```python
from build123d import *

# Parameters (mm, degrees)
SKETCH1_W                  = 19.05
SKETCH1_H                  = 63.5
BOSS_EXTRUDE1_DEPTH        = 15.875
SKETCH2_R                  = 5.1435
CUT_EXTRUDE1_DEPTH         = 37.753282166
SKETCH3_R                  = 12.7
CUT_EXTRUDE2_DEPTH         = 3.96875
SKETCH4_R                  = 12.7
SKETCH4_R_2                = 7.9375
CUT_EXTRUDE3_DEPTH         = 0.79375
F_10_CLEARANCE_HOLE1_D     = 5.6134
F_10_CLEARANCE_HOLE1_DEPTH = 25.4
F_10_CLEARANCE_HOLE1_TIP   = 1.686435499
FILLET1_R                  = 1.5875
BOSS_EXTRUDE2_DEPTH        = 5.953125
FILLET3_R                  = 0.79375
FILLET4_R                  = 3.175


with BuildPart() as part:
    # Sketch1 → Boss-Extrude1 (new body)
    with BuildSketch(Plane.XY):
        Rectangle(SKETCH1_W, SKETCH1_H)
    extrude(amount=BOSS_EXTRUDE1_DEPTH)

    # Sketch2 → Cut-Extrude1 (cut, through all)
    with BuildSketch(Plane.XY.offset(15.875)):
        Circle(SKETCH2_R)
    extrude(amount=-CUT_EXTRUDE1_DEPTH, mode=Mode.SUBTRACT)

    # Sketch3 → Cut-Extrude2 (cut)
    with BuildSketch(Plane.XY.offset(15.875)):
        Circle(SKETCH3_R)
    extrude(amount=-CUT_EXTRUDE2_DEPTH, mode=Mode.SUBTRACT)

    # Sketch4 → Cut-Extrude3 (cut)
    with BuildSketch(Plane.XY.offset(11.90625)):
        Circle(SKETCH4_R)
        Circle(SKETCH4_R_2, mode=Mode.SUBTRACT)
    extrude(amount=-CUT_EXTRUDE3_DEPTH, mode=Mode.SUBTRACT)

    # #10 Clearance Hole1
    with Locations(Plane.XY.offset(15.875)):
        with Locations((0, 25.4), (0, -25.4)):
            Hole(F_10_CLEARANCE_HOLE1_D / 2, depth=F_10_CLEARANCE_HOLE1_DEPTH)
            with Locations((0, 0, -(F_10_CLEARANCE_HOLE1_DEPTH + F_10_CLEARANCE_HOLE1_TIP / 2))):  # 118° drill point
                Cone(0, F_10_CLEARANCE_HOLE1_D / 2, F_10_CLEARANCE_HOLE1_TIP, mode=Mode.SUBTRACT)

    # Fillet1
    fillet1_edges = [part.edges().sort_by_distance(p)[0] for p in [
        (9.525, -8.400260413, 13.49375),
        (-9.525, -8.400260413, 13.49375),
        (9.525, 8.400260413, 13.49375),
        (-9.525, 8.400260413, 13.49375),
        (-9.525, 0, 11.1125),
        (9.525, 0, 11.1125),
        (9.525, -31.75, 7.9375),
        (-9.525, -31.75, 7.9375),
    ]]
    fillet(fillet1_edges, radius=FILLET1_R - 0.0001)  # a hair under: the kernel refuses the full size

    # Sketch12 → Boss-Extrude2 (add)
    with BuildSketch(Plane(origin=(0, 0, 0), x_dir=(-1, 0, 0), z_dir=(0, 0, -1))):
        with BuildLine():
            Line((-15.875, 67.31), (-15.875, 51.435))
            Line((-15.875, 51.435), (-9.779, 51.435))
            Line((-9.779, 51.435), (-9.779, 54.61))
            ThreePointArc((-9.779, 54.61), (-6.604, 57.785), (-3.429, 54.61))
            Line((-3.429, 54.61), (-3.429, 45.085))
            Line((-3.429, 45.085), (-15.875, 45.085))
            Line((-15.875, 45.085), (-15.875, 31.75))
            Line((-15.875, 31.75), (-9.525, 3.175))
            Line((-9.525, 3.175), (-9.525, 31.75))
            Line((-9.525, 31.75), (9.525, 31.75))
            Line((9.525, 31.75), (9.525, 67.31))
            Line((9.525, 67.31), (-15.875, 67.31))
        make_face()
    extrude(amount=-BOSS_EXTRUDE2_DEPTH)

    # Fillet3
    fillet3_edges = [part.edges().sort_by_distance(p)[0] for p in [
        (9.779, 51.435, 2.9765625),
        (15.875, 51.435, 2.9765625),
        (9.525, 3.175, 2.9765625),
        (15.875, 31.75, 2.9765625),
        (15.875, 45.085, 2.9765625),
        (3.429, 45.085, 2.9765625),
    ]]
    fillet(fillet3_edges, radius=FILLET3_R)

    # Fillet4
    fillet4_edges = [part.edges().sort_by_distance(p)[0] for p in [
        (15.875, 67.31, 2.9765625),
        (-9.525, 67.31, 2.9765625),
    ]]
    fillet(fillet4_edges, radius=FILLET4_R)


with BuildPart() as body_2:
    # Mirror1: mirrored copy
    add(part.part.mirror(Plane.XY.offset(15.875)))


solid = body_2.part
```
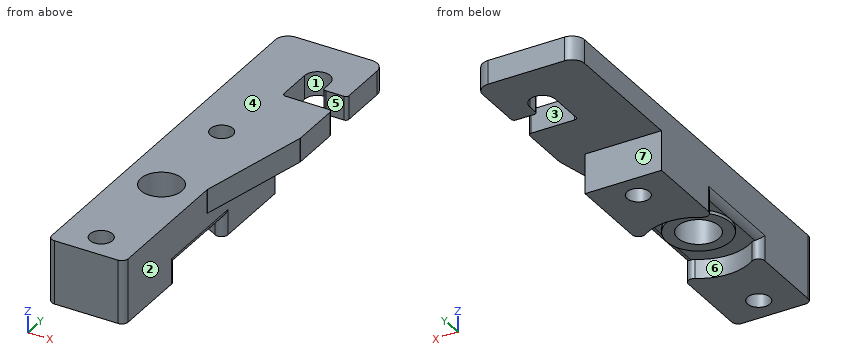
Design review of the part built by this model. Coordinates are the model's own, in mm. Face numbers are marked on the shaded views. A direction names the side the tool comes from. Give positions to 0.01 mm unless a question says otherwise; leave off trailing zeros. Order: outer loops, then holes, each group sorted by start corner. A loop starts at its lowest first (then second) coordinate and runs counter-clockwise, first axis right, second up. Notation, with made-up numbers: (54, 39) -> (96, 39) arc R21 ccw to (96, 54) -> close; hole circle Ø10 at (-7.75, 30). An arc over 180 degrees is marked (long way). Write each question's results on one line, items separated by ' | '. Start each with the question number.
Q1. For pin 1 (6.5 mm diameter, centred on x = 0, y = 25.4, fed in from -Z) (3 decimals); pin 2 (4.5 mm diameter, centred on x = 0, y = -25.4, fed in from +Z); pin 3 (3 mm diameter, centred on x = -1.5, z = 20, fed in from +Y); pin 4 (8 mm diameter, centred on y = 2.5, z = 22.5, fed in from +X), all flat-tipped, find the tip position at first contact; note any pin that passes through.
Q2. Add section B-B on x = 0. State how many separate pieces and enclosed holes the cut face has, and give its area (3 significant figures).
Q3. Add section A-A on z = 18. Give the boundary of the cut face in (x, y) (3 decimals).
Q4. Wall thickness on L1, parallel to Y at x = 0, z = 25; L2, parallel to Y at x = 0, z = 20; L3, parallel to Y at x = 0, z = 26.5: over which ranges is each line inside the solid? List them lowest first. Write a range as from..to.
Q5. Mouldability with a two-part tool opening along X and no side actions: class the marked faces 1, 2 and 3 as +X half, -X half, draft (parallel to the pull), parting line (faces both ways), or undercut.
Q6. Add section C-C on y = -25.4. Give the boundary of the cut face in (x, z) (3 decimals).
Q7. Machinability: for the marked faces 4, 5, 6 and 7, which of the approach directions +Z, -Z, +X, -X, +Y, -Y give a long, thin tool a straight path to every point of the face, cutting with its end or side? Answer none if there is none.
Found:
1) pin 1: stops at z = 15.875 | pin 2: passes through | pin 3: stops at y = 31.75 | pin 4: stops at x = 9.88
2) separate pieces: 4 | enclosed holes: 0 | area: 811 mm2
3) outline: (-9.525, -30.163) arc R1.587 ccw to (-7.938, -31.75) -> (7.938, -31.75) arc R1.587 ccw to (9.525, -30.163) -> (9.525, -11.88) arc R1.587 ccw to (7.056, -10.56) arc R12.7 cw to (-7.056, -10.56) arc R1.587 ccw to (-9.525, -11.88) -> close; (-9.525, 11.88) arc R1.587 ccw to (-7.056, 10.56) arc R12.7 cw to (7.056, 10.56) arc R1.587 ccw to (9.525, 11.88) -> (9.525, 31.75) -> (-9.525, 31.75) -> close; hole circle Ø5.613 at (0, -25.4); hole circle Ø5.613 at (0, 25.4)
4) L1: y = -31.75..-28.21, -22.59..-5.14, 5.14..22.59, 28.21..31.75 | L2: y = -31.75..-28.21, -22.59..-12.7, -7.94..-5.14, 5.14..7.94, 12.7..22.59, 28.21..31.75 | L3: y = -31.75..-28.21, -22.59..-5.14, 5.14..22.59, 28.21..67.31
5) face 1: undercut | face 2: +X half | face 3: draft
6) outline: (-9.525, 15.875) -> (-2.807, 15.875) -> (-2.807, 31.75) -> (-9.525, 31.75) -> close; (2.807, 15.875) -> (9.525, 15.875) -> (9.525, 31.75) -> (2.807, 31.75) -> close
7) face 4: +Z, +X, -X, +Y, -Y | face 5: +Z, -Z, +X | face 6: -Z | face 7: -Z, +X, -X, +Y
